from build123d import *

# Parameters (mm, degrees)
F0_W     = 127
F0_H     = 127
F1_DEPTH = 101.6
F3_DEPTH = 76.2
F4_R     = 6.35
F5_DEPTH = 203.2
F6_T     = -2.54
F7_R     = 5.08


with BuildPart() as f1:
    # F0 (on Top) → F1 (new body)
    with BuildSketch(Plane.XY):
        Rectangle(F0_W, F0_H)
    extrude(amount=F1_DEPTH)

    # F2 (on face) → F3 (cut)
    with BuildSketch(Plane.XY.offset(101.6)):
        Polygon((63.5, -63.5), (63.5, -12.7), (12.7, -63.5), align=None)
        Polygon((-63.5, 12.7), (-12.7, 63.5), (-63.5, 63.5), align=None)
    extrude(amount=-F3_DEPTH, mode=Mode.SUBTRACT)

    # F4 (on face) → F5 (cut)
    with BuildSketch(Plane.XY.offset(25.4)):
        with Locations((-47.3392494023, 48.0060018599)):
            Circle(F4_R)
        with Locations((47.9774476191, -47.1440458012)):
            Circle(F4_R)
    extrude(amount=-F5_DEPTH, mode=Mode.SUBTRACT)

    # F6
    f6_openings = [f1.faces().sort_by_distance(p)[0] for p in [
        (-0.005092, -0.006878, 0),
    ]]
    offset(amount=F6_T, openings=f6_openings, kind=Kind.INTERSECTION)

    # F7
    f7_edges = [f1.edges().sort_by_distance(p)[0] for p in [
        (-38.1, 38.1, 101.6),
        (-63.5, -25.4, 101.6),
        (-63.5, 12.7, 63.5),
        (25.4, 63.5, 101.6),
        (63.5, 25.4, 101.6),
        (38.1, -38.1, 101.6),
        (63.5, -12.7, 63.5),
        (12.7, -63.5, 63.5),
        (-25.4, -63.5, 101.6),
        (63.5, -38.1, 25.4),
        (38.1, -63.5, 25.4),
        (63.5, 63.5, 50.8),
        (-12.7, 63.5, 63.5),
        (-38.1, 63.5, 25.4),
        (-63.5, 38.1, 25.4),
        (-63.5, -63.5, 50.8),
    ]]
    fillet(f7_edges, radius=F7_R)


solid = f1.part
Model file for the job. Use its own axes, mm. A direction names the side the tool comes from. Give positions to 0.01 mm unless a question says otherwise; leave off trailing zeros. Loops run counter-clockwise (first coordinate to the right, second up) from the corner with the lowest first, then second, coordinate; pieces in that order, holes last. Notation, with made-up numbers: (-19, 71.25) -> (28, 71.25) arc R19 ccw to (28, 85.25) -> close; hole circle Ø8 at (26, 29.5). An arc over 180 degrees is marked (long way). Use a Markdown table: item, result. Add a question column.
(1) Drop flat-ended pins along their axis: pin 1 Ø15 at (x, y) = (25, -47.5) entering from -Z; pin 2 Ø6 at (x, y) = (-15, -36) entering from -Z; pin 3 Ø3 at (y, z) = (41, 25.5) entering from -X. Give the stop position or say it passes through.
(2) Wall check: line 1 along X through (y, z) = (0.5, 36); line 2 along Y through (x, z) = (-48.5, 23); line 3 along X through (y, z) = (40, 21). Give the ranges that are in metal, low to high.
(3) Tool access for faces 1 (the flat face through (10, 63.5, 37)), 2 (the flat face through (-60.96, -14, 38)), 3 (the cylindrical face through (-63.124, 12.514, 57.887)), 4 (the cylindrical face through (12.514, -63.124, 57.887)): list every direction of +Z, -Z, +X, -X, +Y, -Y with a clear straight run to the whole face (end or side of a thin tool).
(4) Slice it at A-A on z = 87. List the corners of the cut face in (x, y).
(5) Slice it at B-B on x = 8.5. List the corners of the cut face in (y, z).
(6) Slice it at D-D on z = 10. List the corners of the cut face in (x, y).
Filled sheet:
| question | item | result |
|---|---|---|
| 1 | pin 1 | z = 22.86 |
| 1 | pin 2 | z = 99.06 |
| 1 | pin 3 | x = -61.92 |
| 2 | line 1 | -63.5 to -60.96, 60.96 to 63.5 |
| 2 | line 2 | -63.5 to -60.96, 24.11 to 41.76, 54.25 to 62.74 |
| 2 | line 3 | -63.45 to -60.96, -51.2 to -43.47, 60.96 to 63.5 |
| 3 | face 1 | +Z, -Z, +X, -X, +Y |
| 3 | face 2 | -Z |
| 3 | face 3 | +Z, -X, +Y |
| 3 | face 4 | +Z, +X, -Y |
| 4 | outline | (-63.5, -58.42) arc R5.08 ccw to (-58.42, -63.5) -> (10.6, -63.5) arc R5.08 ccw to (14.19, -62.01) -> (62.01, -14.19) arc R5.08 ccw to (63.5, -10.6) -> (63.5, 58.42) arc R5.08 ccw to (58.42, 63.5) -> (-10.6, 63.5) arc R5.08 ccw to (-14.19, 62.01) -> (-62.01, 14.19) arc R5.08 ccw to (-63.5, 10.6) -> close; hole (-60.96, -60.96) -> (11.65, -60.96) -> (60.96, -11.65) -> (60.96, 60.96) -> (-11.65, 60.96) -> (-60.96, 11.65) -> close |
| 5 | outline | (-63.5, 0) -> (-60.96, 0) -> (-60.96, 99.06) -> (60.96, 99.06) -> (60.96, 0) -> (63.5, 0) -> (63.5, 96.52) arc R5.08 ccw to (58.42, 101.6) -> (-58.42, 101.6) arc R5.08 ccw to (-63.5, 96.52) -> close |
| 6 | outline | (-63.5, -58.42) arc R5.08 ccw to (-58.42, -63.5) -> (63.5, -63.5) -> (63.5, 58.42) arc R5.08 ccw to (58.42, 63.5) -> (-63.5, 63.5) -> close; circle Ø17.78 at (-47.34, 48.01); circle Ø17.78 at (47.98, -47.14); hole (-60.96, -60.96) -> (60.96, -60.96) -> (60.96, 60.96) -> (-60.96, 60.96) -> close; hole circle Ø12.7 at (-47.34, 48.01); hole circle Ø12.7 at (47.98, -47.14) |
